from build123d import *

# Parameters (mm, degrees)
ESQUISSE1_W        = 3
ESQUISSE1_H        = 16
BOSS_EXTRU_1_DEPTH = 4


with BuildPart() as part:
    # Esquisse1 → Base-Révolution (revolve)
    with BuildSketch(Plane(origin=(0, 0, 0), x_dir=(1, 0, 0), z_dir=(0, 1, 0))):
        with Locations((1.5, -8)):
            Rectangle(ESQUISSE1_W, ESQUISSE1_H)
    revolve(axis=Axis((0, 0, 0), (0, 0, 1)))

    # Chanfrein1: read off the stored shape, not the designer's step
    # Chanfrein1 outline → Chanfrein1 (revolve, cut)
    with BuildSketch(Plane.XZ):
        Polygon((3, 16), (2.4, 16), (3, 15.4), align=None)
    revolve(axis=Axis((0, 0, 0), (0, 0, 1)), mode=Mode.SUBTRACT)

    # Esquisse6 → Boss.-Extru.1 (add)
    with BuildSketch(Plane.XY):
        Polygon((5, -2.886751346), (5, 2.886751346), (0, 5.773502692), (-5, 2.886751346), (-5, -2.886751346), (0, -5.773502692), align=None)
    extrude(amount=-BOSS_EXTRU_1_DEPTH)

    # Esquisse7 → Enlèvement de matière-Révolution1 (revolve, cut)
    with BuildSketch(Plane(origin=(0, 0, 0), x_dir=(1, 0, 0), z_dir=(0, 1, 0))):
        Polygon((-5, 4), (-11.92820323, 4), (-11.92820323, 0), align=None)
    revolve(axis=Axis((0, 0, -6.239446496), (0, 0, 1)), mode=Mode.SUBTRACT)


solid = part.part
Verification items for the finished model (mm, model axes). A direction names the side the tool comes from. Coordinates: 2 decimals unless noted, no trailing zeros. Loops run counter-clockwise (first coordinate to the right, second up) from the corner with the lowest first, then second, coordinate; pieces in that order, holes last. Notation, with made-up numbers: M -21.5,52.25 L 20.5,52.25 A4 cw 20.5,56.25 Z; hole C -25.75,66.25 d5. An arc over 180 degrees is marked long. One line per item, written item: value.
1. Section check A-A on z = -1.75. Record the cut outline in (x, y), plus the area to 3 significant figures.
Answers follow:
outline: M -5,-2.89 L 0,-5.77 L 5,-2.89 L 5,2.89 L 0,5.77 L -5,2.89 Z
area: 86.6 mm^2
2. Gauge pin test, flat ends, axial feed: P1, Ø3, axis at x = -3, z = 13.5, coming from the +Y side; P2, Ø5, axis at y = -2, z = 8, coming from the -X side; P3, Ø1.5, axis at x = -1.5, z = -1, coming from the +Y side. Record the tip position at first contact, or that the pin passes through.
Answers follow:
P1: y = 2.6
P2: x = -3
P3: y = 5.34
3. Section check B-B on z = 9.25. Record the cut outline in (x, y).
Answers follow:
outline: C 0,0 d6
4. Set-up check for faces 1 (the conical face through (4.483, -2.603, -3.894)), 2 (the flat face through (2.2, -2.5, 0)): record each of +Z, -Z, +X, -X, +Y, -Y from which the full face is reachable in a straight line by a thin tool's end or side.
Answers follow:
face 1: -Z, +X, -Y
face 2: +Z
5. Material ranges on line 1 along Z through (x, y) = (4.5, -1.25); line 2 along Y through (x, z) = (-1, 14.75); line 3 along Y through (x, z) = (1.25, 9), recorded low to high. Write a range as from..to.
Answers follow:
line 1: -4..0
line 2: -2.83..2.83
line 3: -2.73..2.73
